```python
from build123d import *

# Parameters (mm, degrees)
SKETCH1_W           = 30
SKETCH1_H           = 25
BOSS_EXTRUDE1_DEPTH = 20
SKETCH2_R           = 5.25
CUT_EXTRUDE1_DEPTH  = 15
CUT_EXTRUDE2_REACH  = 29.951
SKETCH3_R           = 2.75
SKETCH4_R           = 2.65
BOSS_EXTRUDE2_DEPTH = 6
CHAMFER1_SIZE       = 8
CHAMFER1_SIZE2      = 13.856406461
SKETCH5_W           = 10
SKETCH5_H           = 19
CUT_EXTRUDE3_DEPTH  = 20
CHAMFER2_SIZE       = 2


with BuildPart() as part:
    # Sketch1 → Boss-Extrude1 (new body)
    with BuildSketch(Plane.XY):
        Rectangle(SKETCH1_W, SKETCH1_H)
    extrude(amount=BOSS_EXTRUDE1_DEPTH)

    # Sketch2 → Cut-Extrude1 (cut)
    with BuildSketch(Plane.XY):
        with Locations((0, 4)):
            Circle(SKETCH2_R)
    extrude(amount=CUT_EXTRUDE1_DEPTH, mode=Mode.SUBTRACT)

    # Sketch3 → Cut-Extrude2 (cut, up to next)
    with BuildSketch(Plane.XY, mode=Mode.PRIVATE) as cut_extrude2_sk1:
        with Locations((0, 4)):
            Circle(SKETCH3_R)
    cut_extrude2_tool1 = extrude(cut_extrude2_sk1.sketch, amount=CUT_EXTRUDE2_REACH, mode=Mode.PRIVATE) & part.part
    add(cut_extrude2_tool1.solids().sort_by_distance((0, 4, 0))[0], mode=Mode.SUBTRACT)

    # Sketch4 → Boss-Extrude2 (add)
    # profile 1 of 2: a face of its own
    with BuildSketch(Plane.XZ.offset(12.5)):
        with BuildLine():
            Line((-15, 20), (-24.395973154, 16.577181208))
            ThreePointArc((-24.395973154, 16.577181208), (-29, 10), (-24.395973154, 3.422818792))
            Line((-24.395973154, 3.422818792), (-15, 0))
            Line((-15, 0), (-15, 20))
        make_face()
        with Locations(Location((-22, 10, 0), (0, 0, 270))):
            Circle(SKETCH4_R, mode=Mode.SUBTRACT)
    # profile 2 of 2: a face of its own
    with BuildSketch(Plane.XZ.offset(12.5)):
        with BuildLine():
            Line((15, 0), (24.395973154, 3.422818792))
            ThreePointArc((24.395973154, 3.422818792), (29, 10), (24.395973154, 16.577181208))
            Line((24.395973154, 16.577181208), (15, 20))
            Line((15, 20), (15, 0))
        make_face()
        with Locations(Location((22, 10, 0), (0, 0, 90))):
            Circle(SKETCH4_R, mode=Mode.SUBTRACT)
    extrude(amount=-BOSS_EXTRUDE2_DEPTH)

    # Chamfer1
    chamfer1_edges = [part.edges().sort_by_distance(p)[0] for p in [
        (-15, 12.5, 10),
        (15, 12.5, 10),
    ]]
    chamfer1_side = [part.faces().sort_by_distance(p)[0] for p in [
        (0, 12.5, 10),
    ]]
    chamfer(chamfer1_edges, length=CHAMFER1_SIZE, length2=CHAMFER1_SIZE2, reference=chamfer1_side[0])

    # Sketch5 → Cut-Extrude3 (cut, symmetric)
    with BuildSketch(Plane(origin=(0, 0, 0), x_dir=(0, 0, -1), z_dir=(1, 0, 0))):
        with Locations((-5, 3)):
            Rectangle(SKETCH5_W, SKETCH5_H)
    extrude(amount=CUT_EXTRUDE3_DEPTH, both=True, mode=Mode.SUBTRACT)

    # Chamfer2
    chamfer2_edges = [part.edges().sort_by_distance(p)[0] for p in [
        (-15, -6.5, 15),
        (15, -6.5, 15),
        (0, -6.5, 10),
    ]]
    chamfer(chamfer2_edges, length=CHAMFER2_SIZE)


solid = part.part
```
Geometry: final body of the model. Coordinates: model frame, mm. A direction names the side the tool comes from. Round coordinates to 2 decimals unless told otherwise and drop trailing zeros. Order: outer loops, then holes, each group sorted by start corner. A loop starts at its lowest first (then second) coordinate and runs counter-clockwise, first axis right, second up. Notation, with made-up numbers: M 31.5,29 L 63.5,29 A19 cw 63.5,52 Z; hole C -13,23 d7. An arc over 180 degrees is marked long. Use one line per item in the form item = value. Start each with the question number.
Q1. Access query for faces 4 (the face through (-0.4, -6.5, 7.6)), 5 (the face through (15, -3, 15)), 6 (the face through (4, 0, 10)). Directions: +Z, -Z, +X, -X, +Y, -Y. A direction counts if a zero-diameter tool reaches every point of the face in a straight line with its end or side. Return the directions, or none.
Q2. Cut plane A-A (x = 0). Return loops of the section in (y, z), and give its area (3 significant figures).
Q3. Cut plane D-D (y = 4). Return loops of the section in (x, z).
Q4. Cut plane C-C (x = 6). Return loops of the section in (y, z).
Q5. Material intervals for line 1 (X direction, y = -7.75, z = 10.25); line 2 (Z direction, x = 10, y = 1.75); line 3 (Y direction, x = 0, z = 12.9), sorted ascending. Write a range as [from, to].
Q6. Cut plane B-B (z = 18). Return loops of the section in (x, y).
Q7. Pin query (flat end, axial travel): pin 1 Ø0.9 at (y, z) = (-3.5, 13.5) entering from -X; pin 2 Ø5 at (x, z) = (22, 10) entering from -Y; pin 3 Ø12 at (x, y) = (0, 4) entering from -Z; pin 4 Ø5 at (x, y) = (-2, 5.5) entering from -Z. Return the tip coordinate at first contact, or that it passes through.
Q8. Mould query, pull axis Z, two halves, no side actions, for faces 1 (the face through (21.883, -9.542, 7.353)), 2 (the face through (19.632, -9.542, 1.687)), 3 (the face through (0, -3, 20)). Classes: +Z half, -Z half, draft (parallel to the pull), parting line (faces both ways), or undercut.
Geometry results:
q1.face_4 = -Z, +Y
q1.face_5 = +Z, -Z, +X, +Y
q1.face_6 = -Z, +X, -X, +Y
q2.outline = M -12.5,0 L -6.5,0 L -6.5,8 L -4.5,10 L -1.25,10 L -1.25,15 L 1.25,15 L 1.25,20 L -12.5,20 Z; M 6.75,15 L 9.25,15 L 9.25,10 L 12.5,10 L 12.5,20 L 6.75,20 Z
q2.area = 232 mm^2
q3.outline = M -11.91,10 L -5.25,10 L -5.25,15 L -2.75,15 L -2.75,20 L -11.91,20 Z; M 2.75,15 L 5.25,15 L 5.25,10 L 11.91,10 L 11.91,20 L 2.75,20 Z
q4.outline = M -12.5,0 L -6.5,0 L -6.5,8 L -4.5,10 L 12.5,10 L 12.5,20 L -12.5,20 Z
q5.line_1 = [-29, -24.64], [-19.36, 19.36], [24.64, 29]
q5.line_2 = [10, 20]
q5.line_3 = [-12.5, -1.25], [9.25, 12.5]
q6.outline = M -20.49,-12.5 L 20.49,-12.5 L 20.49,-6.5 L 17,-6.5 L 15,-4.5 L 15,-1.36 L 7,12.5 L -7,12.5 L -15,-1.36 L -15,-4.5 L -17,-6.5 L -20.49,-6.5 Z; hole C 0,4 d5.5
q7.pin_1 = -15
q7.pin_2 = through
q7.pin_3 = 10
q7.pin_4 = 15
q8.face_1 = undercut
q8.face_2 = -Z half
q8.face_3 = +Z half
